Here's the drawing with two shaded views (mm, measured from the low corner). I have some questions. A direction names the side the tool comes from. Give positions to 0.01 mm unless a question says otherwise; leave off trailing zeros. Write each loop counter-clockwise with the first axis right and the second up, starting at its lowest first coordinate (ties: lowest second). Pieces come first, ordered by that corner, then holes. Notation, with made-up numbers: (45, 44) - (49, 44) arc R21 ccw to (49, 76) - close; hole circle Ø5 at (60.5, 1). An arc over 180 degrees is marked (long way). Use one line per item in the form item = value.
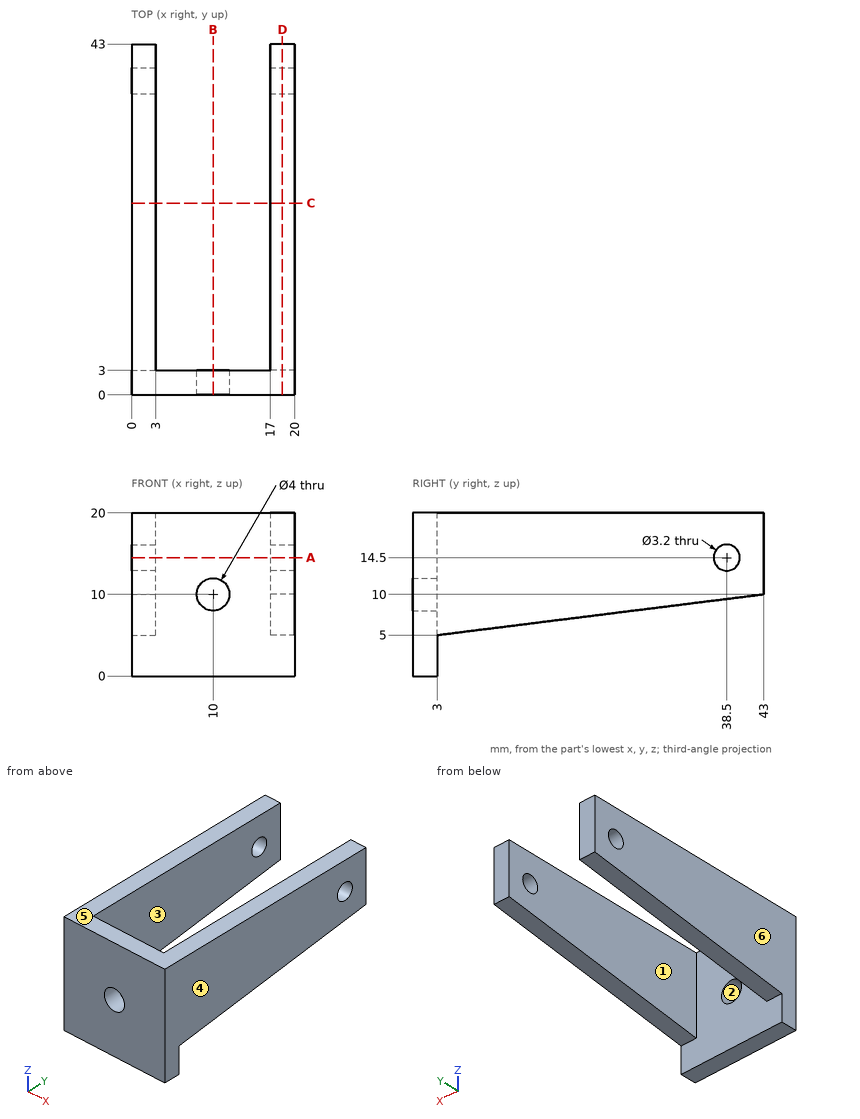
1. Imagine slicing it at B-B, the plane x = 10. List the corners of the cut face in (y, z) for me.
Response values:
outline = (0, 0) - (3, 0) - (3, 8) - (0, 8) - close; (0, 12) - (3, 12) - (3, 20) - (0, 20) - close
2. Imagine slicing it at D-D, the plane x = 18.5. List the corners of the cut face in (y, z) for me.
Response values:
outline = (0, 0) - (3, 0) - (3, 5) - (43, 10) - (43, 20) - (0, 20) - close; hole circle Ø3.2 at (38.5, 14.5)
3. If we mould it in two halves opening along X, with no side actions, what happens to the marked faces 3, 4, 5 and 6? For each: pulls with the +X half, pulls with the -X half, needs draft (parallel to the pull), parting line crosses it, or undercut.
Response values:
face_3 = undercut
face_4 = pulls with the +X half
face_5 = needs draft
face_6 = pulls with the -X half
4. For pin 1 (10 mm diameter, centred on x = 10.5, y = 17.5, fed in from +Z); pin 2 (6 mm diameter, centred on x = 5.5, y = 22.5, fed in from -Z), each with a flat end and sliding along its axis, tell me the tip position at first contact or that it passes through.
Response values:
pin_1 = through
pin_2 = 7.23
5. Imagine slicing it at A-A, the plane z = 14.5. List the corners of the cut face in (x, y) for me, and give its area (3 significant figures).
Response values:
outline = (0, 0) - (20, 0) - (20, 36.9) - (17, 36.9) - (17, 3) - (3, 3) - (3, 36.9) - (0, 36.9) - close; (0, 40.1) - (3, 40.1) - (3, 43) - (0, 43) - close; (17, 40.1) - (20, 40.1) - (20, 43) - (17, 43) - close
area = 281 mm²
6. Imagine slicing it at C-C, the plane y = 23.5. List the corners of the cut face in (x, z) for me, and give its area (3 significant figures).
Response values:
outline = (0, 7.56) - (3, 7.56) - (3, 20) - (0, 20) - close; (17, 7.56) - (20, 7.56) - (20, 20) - (17, 20) - close
area = 74.6 mm²
7. If I drill on line 1 (X direction, y = 15, z = 11); line 2 (X direction, y = 0.8, z = 10), over which ranges is the centre line in solid material (lowest first)? Write a range as from..to.
Response values:
line_1 = 0..3, 17..20
line_2 = 0..8, 12..20
8. Which directions (+Z, -Z, +X, -X, +Y, -Y) give clear straight access to the entire face, cutting with the end or side of a thin tool? Please do the marked faces 1 and 2.
Response values:
face_1 = +Z, -Z, +Y
face_2 = +Y, -Y
